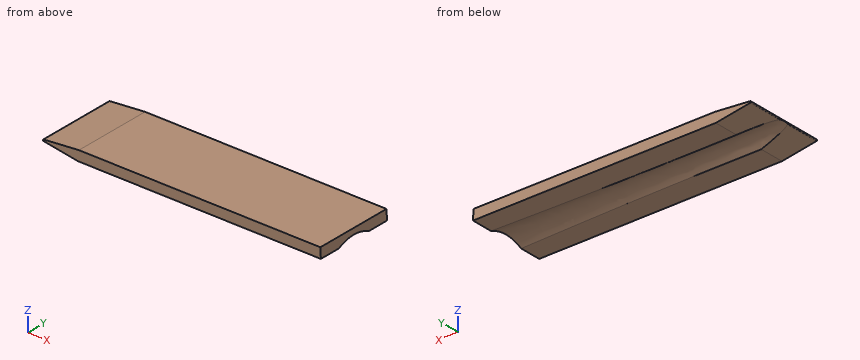
```python
from build123d import *

# Parameters (mm, degrees)
BOSS_EXTRUDE1_DEPTH = 80


with BuildPart() as part:
    # Sketch1 → Boss-Extrude1 (new body)
    with BuildSketch(Plane(origin=(0, 0, 0), x_dir=(1, 0, 0), z_dir=(0, 1, 0))):
        with BuildLine():
            Line((180, 5), (179.469862502, -5.115626071))
            Line((179.469862502, -5.115626071), (-63.767328769, -5.115626071))
            Line((-63.767328769, -5.115626071), (-99.406651233, -1.997589379))
            ThreePointArc((-99.406651233, -1.997589379), (-99.829230269, -1.789196461), (-100, -1.350062826))
            Line((-100, -1.350062826), (-100, -1.154739941))
            ThreePointArc((-100, -1.154739941), (-99.844263878, -0.732598709), (-99.451682402, -0.512742519))
            Line((-99.451682402, -0.512742519), (-64.645595971, 5))
            Line((-64.645595971, 5), (180, 5))
        make_face()
    extrude(amount=BOSS_EXTRUDE1_DEPTH)

    # Cut-Loft2: read off the stored shape, not the designer's step
    # Cut-Loft2: loft between two sections, ruled curve by curve
    cut_loft2_from = [
        Edge.make_bspline([(-100, 46.372269689, -42.924050086), (-100, 47.27138594, -42.658538849), (-100, 48.210787476, -42.320500231), (-100, 50.149850676, -41.453921439), (-100, 51.149765287, -40.925166444), (-100, 53.169114931, -39.628159499), (-100, 54.18874158, -38.859470423), (-100, 56.178772716, -37.039694285), (-100, 57.149111753, -35.987936251), (-100, 58.941067781, -33.581924282), (-100, 59.762113682, -32.226944596), (-100, 61.133842388, -29.23911219), (-100, 61.683362519, -27.605929091), (-100, 62.216554733, -25.013126268), (-100, 62.345428507, -24.125166051), (-100, 62.496577402, -22.320181761), (-100, 62.518852521, -21.403157688), (-100, 62.447919377, -19.558367046), (-100, 62.354526015, -18.630982172), (-100, 62.052716958, -16.78785196), (-100, 61.844301264, -15.872106621), (-100, 61.313278789, -14.073874119), (-100, 60.990797696, -13.191812573), (-100, 60.242941855, -11.480401071), (-100, 59.817567108, -10.651051116), (-100, 58.87497002, -9.063664977), (-100, 58.358110433, -8.305848706), (-100, 57.250681403, -6.872525569), (-100, 56.660111959, -6.197018701), (-100, 54.80395718, -4.309795913), (-100, 53.45539094, -3.237122381), (-100, 50.680622933, -1.473760637), (-100, 49.255217853, -0.782163442), (-100, 46.443698676, 0.264430993), (-100, 45.057669802, 0.620347796), (-100, 42.398313027, 1.067148265), (-100, 41.124675582, 1.158630823), (-100, 38.724689029, 1.150596935), (-100, 37.597941582, 1.051343402), (-100, 35.499184882, 0.725544061), (-100, 34.526846562, 0.499041204), (-100, 32.72861406, -0.03198127), (-100, 31.789212524, -0.370019888), (-100, 29.850149324, -1.23659868), (-100, 28.850234713, -1.765353674), (-100, 26.830885069, -3.062360619), (-100, 25.81125842, -3.831049696), (-100, 23.821227284, -5.650825833), (-100, 22.850888247, -6.702583867), (-100, 21.058932219, -9.108595836), (-100, 20.237886318, -10.463575522), (-100, 18.866157612, -13.451407929), (-100, 18.316637481, -15.084591028), (-100, 17.783445267, -17.677393851), (-100, 17.654571493, -18.565354067), (-100, 17.503422598, -20.370338357), (-100, 17.481147479, -21.287362431), (-100, 17.552080623, -23.132153073), (-100, 17.645473985, -24.059537946), (-100, 17.947283042, -25.902668159), (-100, 18.155698736, -26.818413497), (-100, 18.686721211, -28.616646), (-100, 19.009202304, -29.498707546), (-100, 19.757058145, -31.210119048), (-100, 20.182432892, -32.039469003), (-100, 21.12502998, -33.626855142), (-100, 21.641889567, -34.384671412), (-100, 22.749318597, -35.81799455), (-100, 23.339888041, -36.493501417), (-100, 25.19604282, -38.380724205), (-100, 26.54460906, -39.453397738), (-100, 29.319377067, -41.216759482), (-100, 30.744782147, -41.908356676), (-100, 33.556301324, -42.954951112), (-100, 34.942330198, -43.310867915), (-100, 37.601686973, -43.757668384), (-100, 38.875324418, -43.849150941), (-100, 41.275310971, -43.841117054), (-100, 42.402058418, -43.74186352), (-100, 44.500815118, -43.416064179), (-100, 45.473153438, -43.189561323), (-100, 46.372269689, -42.924050086)], [0, 0, 0, 0, 0.03125, 0.03125, 0.0625, 0.0625, 0.09375, 0.09375, 0.125, 0.125, 0.15625, 0.15625, 0.1875, 0.1875, 0.203125, 0.203125, 0.21875, 0.21875, 0.234375, 0.234375, 0.25, 0.25, 0.265625, 0.265625, 0.28125, 0.28125, 0.296875, 0.296875, 0.3125, 0.3125, 0.34375, 0.34375, 0.375, 0.375, 0.40625, 0.40625, 0.4375, 0.4375, 0.46875, 0.46875, 0.5, 0.5, 0.53125, 0.53125, 0.5625, 0.5625, 0.59375, 0.59375, 0.625, 0.625, 0.65625, 0.65625, 0.6875, 0.6875, 0.703125, 0.703125, 0.71875, 0.71875, 0.734375, 0.734375, 0.75, 0.75, 0.765625, 0.765625, 0.78125, 0.78125, 0.796875, 0.796875, 0.8125, 0.8125, 0.84375, 0.84375, 0.875, 0.875, 0.90625, 0.90625, 0.9375, 0.9375, 0.96875, 0.96875, 1, 1, 1, 1], 3),
    ]
    cut_loft2_to = [
        Edge.make_bspline([(180, 28.551057955, -78.935198824), (180, 30.147996066, -79.412238075), (180, 31.875323965, -79.820338386), (180, 35.604608971, -80.411256005), (180, 37.607151324, -80.593998796), (180, 41.873728161, -80.621685223), (180, 44.138472267, -80.46616369), (180, 48.868689715, -79.68670829), (180, 51.334716697, -79.061711462), (180, 56.338793625, -77.216810774), (180, 58.876697195, -75.995271668), (180, 63.819442208, -72.875919018), (180, 66.222872399, -70.976485062), (180, 69.533227056, -67.631805591), (180, 70.587261439, -66.435254593), (180, 72.564064486, -63.89331443), (180, 73.486743413, -62.547940775), (180, 75.171328923, -59.731199346), (180, 75.933152653, -58.259880816), (180, 77.272256632, -55.221524011), (180, 77.849475409, -53.654564318), (180, 78.803553913, -50.460688096), (180, 79.18038475, -48.83386828), (180, 79.727221351, -45.558844421), (180, 79.897235414, -43.910739803), (180, 80.033641397, -40.631524344), (180, 80.000075583, -39.000500123), (180, 79.741415418, -35.790779731), (180, 79.516387593, -34.212145749), (180, 78.582975921, -29.599763352), (180, 77.615177464, -26.693271965), (180, 75.193247864, -21.373934955), (180, 73.741185532, -18.960508489), (180, 70.568939332, -14.673166832), (180, 68.849774783, -12.797964612), (180, 65.322122641, -9.551708587), (180, 63.513755151, -8.179462312), (180, 59.931061785, -5.862405409), (180, 58.156397702, -4.916816601), (180, 54.714031128, -3.36540993), (180, 53.045880155, -2.759208753), (180, 49.852003934, -1.80513025), (180, 48.124676035, -1.39702994), (180, 44.395391029, -0.80611232), (180, 42.392848676, -0.623369529), (180, 38.126271839, -0.595683102), (180, 35.861527733, -0.751204636), (180, 31.131310285, -1.530660035), (180, 28.665283303, -2.155656863), (180, 23.661206375, -4.000557551), (180, 21.123302805, -5.222096657), (180, 16.180557792, -8.341449307), (180, 13.777127601, -10.240883263), (180, 10.466772944, -13.585562734), (180, 9.412738561, -14.782113732), (180, 7.435935514, -17.324053895), (180, 6.513256587, -18.66942755), (180, 4.828671077, -21.486168979), (180, 4.066847347, -22.957487509), (180, 2.727743368, -25.995844314), (180, 2.150524591, -27.562804007), (180, 1.196446087, -30.756680229), (180, 0.81961525, -32.383500046), (180, 0.272778649, -35.658523904), (180, 0.102764586, -37.306628522), (180, -0.033641397, -40.585843981), (180, -7.5583e-05, -42.216868202), (180, 0.258584582, -45.426588594), (180, 0.483612407, -47.005222577), (180, 1.417024079, -51.617604973), (180, 2.384822536, -54.52409636), (180, 4.806752136, -59.84343337), (180, 6.258814468, -62.256859836), (180, 9.431060668, -66.544201493), (180, 11.150225217, -68.419403713), (180, 14.677877359, -71.665659739), (180, 16.486244849, -73.037906013), (180, 20.068938215, -75.354962916), (180, 21.843602298, -76.300551724), (180, 25.285968872, -77.851958395), (180, 26.954119845, -78.458159572), (180, 28.551057955, -78.935198824)], [0, 0, 0, 0, 0.03125, 0.03125, 0.0625, 0.0625, 0.09375, 0.09375, 0.125, 0.125, 0.15625, 0.15625, 0.1875, 0.1875, 0.203125, 0.203125, 0.21875, 0.21875, 0.234375, 0.234375, 0.25, 0.25, 0.265625, 0.265625, 0.28125, 0.28125, 0.296875, 0.296875, 0.3125, 0.3125, 0.34375, 0.34375, 0.375, 0.375, 0.40625, 0.40625, 0.4375, 0.4375, 0.46875, 0.46875, 0.5, 0.5, 0.53125, 0.53125, 0.5625, 0.5625, 0.59375, 0.59375, 0.625, 0.625, 0.65625, 0.65625, 0.6875, 0.6875, 0.703125, 0.703125, 0.71875, 0.71875, 0.734375, 0.734375, 0.75, 0.75, 0.765625, 0.765625, 0.78125, 0.78125, 0.796875, 0.796875, 0.8125, 0.8125, 0.84375, 0.84375, 0.875, 0.875, 0.90625, 0.90625, 0.9375, 0.9375, 0.96875, 0.96875, 1, 1, 1, 1], 3),
    ]
    cut_loft2 = Solid(Shell([*[Face.make_surface_from_curves(cut_loft2_from[k], cut_loft2_to[k]) for k in range(1)], Face(Wire(cut_loft2_from)), Face(Wire(cut_loft2_to))]))
    add(cut_loft2, mode=Mode.SUBTRACT)


solid = part.part
```
Check sheet for the modelled part. Datum: model origin and axes. Units: mm. Round coordinates to 2 decimals unless told otherwise and drop trailing zeros. Write each loop counter-clockwise with the first axis right and the second up, starting at its lowest first coordinate (ties: lowest second). Pieces come first, ordered by that corner, then holes. Notation, with made-up numbers: (-36, 65) -> (-9, 65) arc R19 cw to (-9, 87) -> close; hole circle Ø9 at (67, 87.25). An arc over 180 degrees is marked (long way). One line per question, with ' | ' between items. Start each with the question number.
1. Scan lines: line 1 along Y through (x, z) = (-68.5, -3); line 2 along Z through (x, y) = (-85.5, 63.5); line 3 along X through (y, z) = (39.5, 1.5). Record each from-to range of solid material in increasing order. Write a range as from..to.
2. Sectioned sample at A-A, the plane y = 66. Record the cut outline in (x, z), then the cut area to 3 significant figures.
3. Depth check by flat-ended pin: pin 1 (6 mm diameter, centred on x = 60, y = 41.5, fed in from -Z); pin 2 (3 mm diameter, centred on y = 37.5, z = 2.5, fed in from +X); pin 3 (5 mm diameter, centred on x = 112.5, y = 47, fed in from -Z). Enter the tip coordinate at first touch or a pass-through.
Taken from the geometry:
1) line 1: y = 0..27.8, 52.2..80 | line 2: z = -1.7..3.21 | line 3: x = -99.98..179.66
2) outline: (-100, 1.15) arc R0.65 ccw to (-99.45, 0.51) -> (-64.65, -5) -> (180, -5) -> (179.47, 5.12) -> (-63.77, 5.12) -> (-99.41, 2) arc R0.65 ccw to (-100, 1.35) -> close | area: 2,670 mm^2
3) pin 1: stops at z = -1.3 | pin 2: stops at x = 179.69 | pin 3: stops at z = -2.25
